from build123d import *

# Parameters (mm, degrees)
BOSS_EXTRUDE1_DEPTH = 5.8
SKETCH2_R           = 0.79375
CUT_EXTRUDE1_DEPTH  = 28.558029683
SKETCH3_R           = 6.35
CUT_EXTRUDE2_DEPTH  = 12.7
FILLET1_R           = 1.5875


with BuildPart() as part:
    # Sketch1 → Boss-Extrude1 (new body)
    with BuildSketch(Plane.XY):
        with BuildLine():
            Line((12.325242086, 19.05), (-12.325242086, 19.05))
            ThreePointArc((-12.325242086, 19.05), (-12.507403955, 12.507403955), (-19.05, 12.325242086))
            Line((-19.05, 12.325242086), (-19.05, -12.325242086))
            ThreePointArc((-19.05, -12.325242086), (-12.507403955, -12.507403955), (-12.325242086, -19.05))
            Line((-12.325242086, -19.05), (12.325242086, -19.05))
            ThreePointArc((12.325242086, -19.05), (12.507403955, -12.507403955), (19.05, -12.325242086))
            Line((19.05, -12.325242086), (19.05, 12.325242086))
            ThreePointArc((19.05, 12.325242086), (12.507403955, 12.507403955), (12.325242086, 19.05))
        make_face()
    extrude(amount=BOSS_EXTRUDE1_DEPTH)

    # Sketch2 → Cut-Extrude1 (cut, through all)
    with BuildSketch(Plane.XY.offset(5.8)):
        with Locations((0, 15.875)):
            Circle(SKETCH2_R)
        with Locations((15.875, 0)):
            Circle(SKETCH2_R)
        with Locations((0, -15.875)):
            Circle(SKETCH2_R)
        with Locations((-15.875, 0)):
            Circle(SKETCH2_R)
    extrude(amount=-CUT_EXTRUDE1_DEPTH, mode=Mode.SUBTRACT)

    # Sketch3 → Cut-Extrude2 (cut)
    with BuildSketch(Plane.XY.offset(5.8)):
        Circle(SKETCH3_R)
    extrude(amount=-CUT_EXTRUDE2_DEPTH, mode=Mode.SUBTRACT)

    # Fillet1
    fillet1_edges = [part.edges().sort_by_distance(p)[0] for p in [
        (-12.325242086, 19.05, 2.9),
        (12.325242086, 19.05, 2.9),
        (19.05, 12.325242086, 2.9),
        (19.05, -12.325242086, 2.9),
        (12.325242086, -19.05, 2.9),
        (-12.325242086, -19.05, 2.9),
        (-19.05, -12.325242086, 2.9),
        (-19.05, 12.325242086, 2.9),
    ]]
    fillet(fillet1_edges, radius=FILLET1_R)


solid = part.part
Here's how the part is built. I have some questions about the finished solid (model axes, mm). Give positions to 0.01 mm unless a question says otherwise; leave off trailing zeros. Order: outer loops, then holes, each group sorted by start corner. A loop starts at its lowest first (then second) coordinate and runs counter-clockwise, first axis right, second up. Notation, with made-up numbers: M -9.5,8 L 8.5,8 A22 ccw 8.5,15 Z; hole C -12.75,85 d4. An arc over 180 degrees is marked long. Answer as a JSON object with one key per item and string values. Group by question number.
1) We'd pull the mould along Y, two halves only. Please class faces 1 (the cylindrical face through (-18.419, 10.994, 2.941)), 2 (the cylindrical face through (-18.45, -10.97, 2.94)), 3 (the cylindrical face through (-12.557, -12.459, 2.859)): pulls with the +Y half, pulls with the -Y half, needs draft (parallel to the pull), parting line crosses it, or undercut.
2) Suppose I cut it at C-C, the plane z = 4.9. Count the separate pieces of the cut face and the enclosed holes in it, plus the area to 3 significant figures.
3) Suppose I cut it at D-D, the plane y = 4. Write out the boundary of the cut face in (x, z), plus the area to 3 significant figures.
4) Please list where these lines run through material, in increasing order: L1, parallel to Y at x = 0, z = 4.25; L2, parallel to X at y = -16, z = 0.7; L3, parallel to X at y = -0.5, z = 2.55. Write a range as [from, to].
5) Suppose I cut it at A-A, the plane x = 0. Write out the boundary of the cut face in (y, z), plus the area to 3 significant figures.
Results found:
{
 "1": {"face 1": "pulls with the +Y half", "face 2": "pulls with the -Y half", "face 3": "undercut"},
 "2": {"separate pieces": "1", "enclosed holes": "5", "area": "1,080 mm²"},
 "3": {"outline": "M -19.05,0 L -4.93,0 L -4.93,5.8 L -19.05,5.8 Z; M 4.93,0 L 19.05,0 L 19.05,5.8 L 4.93,5.8 Z", "area": "164 mm²"},
 "4": {"L1": "[-19.05, -16.67], [-15.08, -6.35], [6.35, 15.08], [16.67, 19.05]", "L2": "[-11.11, -0.78], [0.78, 11.11]", "L3": "[-19.05, -16.49], [-15.26, -6.33], [6.33, 15.26], [16.49, 19.05]"},
 "5": {"outline": "M -19.05,0 L -16.67,0 L -16.67,5.8 L -19.05,5.8 Z; M -15.08,0 L -6.35,0 L -6.35,5.8 L -15.08,5.8 Z; M 6.35,0 L 15.08,0 L 15.08,5.8 L 6.35,5.8 Z; M 16.67,0 L 19.05,0 L 19.05,5.8 L 16.67,5.8 Z", "area": "129 mm²"}
}
